```python
from build123d import *

# Parameters (mm, degrees)
F0_W     = 1651
F0_H     = 304.8
F1_DEPTH = 1270
F2_W     = 762
F2_H     = 304.8
F3_DEPTH = 635
F5_DEPTH = 304.8
F8_DEPTH = 576.58


with BuildPart() as f1:
    # F0 (on Front) → F1 (new body)
    with BuildSketch(Plane.XZ):
        with Locations((671.6712, 66.609716)):
            Rectangle(F0_W, F0_H)
    extrude(amount=F1_DEPTH)

    # F2 (on face) → F3 (join)
    with BuildSketch(Plane.XY.offset(219.009716)):
        with Locations((227.1712, -152.4)):
            Rectangle(F2_W, F2_H)
    extrude(amount=F3_DEPTH)

    # F4 (on face) → F5 (join)
    with BuildSketch(Plane.XY.offset(219.009716)):
        with BuildLine():
            ThreePointArc((1497.1712, -1270), (1946.184006, -1084.012806), (2132.1712, -635))
            ThreePointArc((2132.1712, -635), (1946.184006, -185.987194), (1497.1712, 0))
            Line((1497.1712, 0), (1497.1712, -1270))
        make_face()
    extrude(amount=-F5_DEPTH)

    # F7 (on face) → F8 (cut)
    with BuildSketch(Plane.XY.offset(219.009716)):
        with BuildLine():
            ThreePointArc((1497.1712, -947.168186), (1724.531189, -855.763664), (1819.093947, -629.698992))
            ThreePointArc((1819.093947, -629.698992), (1278.656705, -403.634319), (1497.1712, -947.168186))
        make_face()
    extrude(amount=-F8_DEPTH, mode=Mode.SUBTRACT)


solid = f1.part
```
Geometry check sheet. Reference: the model listing, model coordinates, mm. A direction names the side the tool comes from. Coordinates: 2 decimals unless noted, no trailing zeros. Order: outer loops, then holes, each group sorted by start corner. A loop starts at its lowest first (then second) coordinate and runs counter-clockwise, first axis right, second up. Notation, with made-up numbers: M 19.25,2 L 57.25,2 A19 cw 57.25,22 Z; hole C 76.5,43.5 d6. An arc over 180 degrees is marked long. Answer as a JSON object with one key per item and string values.
Q1. Cross-section at A-A on z = 166. Record the cut outline in (x, y), and give its area (3 significant figures).
Results are:
{"outline": "M -153.83,-1270 L 1497.17,-1270 A635 ccw 1497.17,0 L -153.83,0 Z; hole C 1501.59,-629.7 d635", "area": "2,410,000 mm²"}
Q2. Tool access check on faces 1 (the flat face through (477, 0, 273)), 2 (the flat face through (222, -304.8, 532)), 3 (the flat face through (608.171, -155, 532)). Record the directions out of +Z, -Z, +X, -X, +Y, -Y that give a thin tool (end or side, any length) a straight path to the whole face; none if there is none.
Results are:
{"face 1": "+Z, -Z, +X, -X, +Y", "face 2": "+Z, +X, -X, -Y", "face 3": "+Z, +X, +Y, -Y"}
Q3. Cross-section at B-B on y = -517. Record the cut outline in (x, z).
Results are:
{"outline": "M -153.83,-85.79 L 1204.77,-85.79 L 1204.77,219.01 L -153.83,219.01 Z; M 1798.42,-85.79 L 2121.11,-85.79 L 2121.11,219.01 L 1798.42,219.01 Z"}
Q4. Cross-section at C-C on x = 1380. Record the cut outline in (y, z).
Results are:
{"outline": "M -1270,-85.79 L -922.99,-85.79 L -922.99,219.01 L -1270,219.01 Z; M -336.41,-85.79 L 0,-85.79 L 0,219.01 L -336.41,219.01 Z"}
Q5. Scan lines: line 1 (X direction, y = -242, z = 443.5); line 2 (Z direction, x = 676, y = -386.5); line 3 (Y direction, x = -45.5, z = 316). Record each from-to range of solid material in increasing order.
Results are:
{"line 1": "x = -153.83 to 608.17", "line 2": "z = -85.79 to 219.01", "line 3": "y = -304.8 to 0"}
Q6. Cross-section at D-D on x = 49.5. Record the cut outline in (y, z), and give its area (3 significant figures).
Results are:
{"outline": "M -1270,-85.79 L 0,-85.79 L 0,854.01 L -304.8,854.01 L -304.8,219.01 L -1270,219.01 Z", "area": "581,000 mm²"}
Q7. Depth check by flat-ended pin: pin 1 Ø8 at (x, y) = (928, -154.5) entering from +Z. Enter the tip coordinate at first touch or a pass-through.
Results are:
{"pin 1": "stops at z = 219.01"}
